```python
from build123d import *

# Parameters (mm, degrees)
SKETCH4_R           = 1.25
BOSS_EXTRUDE2_DEPTH = 5
CUT_EXTRUDE2_DEPTH  = 10


with BuildPart() as part:
    # Sketch4 → Boss-Extrude2 (new body)
    with BuildSketch(Plane(origin=(0, 0, 0), x_dir=(1, 0, 0), z_dir=(0, 1, 0))):
        Polygon((82.9, -82.75), (79, -82.75), (79, -86), (79, -88.5), (89, -88.5), (89, -80.85), (82.9, -80.85), align=None)
        with Locations((81.5, -86)):
            Circle(SKETCH4_R, mode=Mode.SUBTRACT)
    extrude(amount=BOSS_EXTRUDE2_DEPTH)

    # Sketch5 → Cut-Extrude2 (cut)
    with BuildSketch(Plane(origin=(89, 0, 0), x_dir=(0, 0, -1), z_dir=(1, 0, 0))):
        with BuildLine():
            ThreePointArc((-84.75, 3.75), (-86, 2.5), (-84.75, 1.25))
            Line((-84.75, 1.25), (-84.75, 3.75))
        make_face()
        with BuildLine():
            Line((-84.75, 3.75), (-84.75, 1.25))
            ThreePointArc((-84.75, 1.25), (-83.866116524, 1.616116524), (-83.5, 2.5))
            ThreePointArc((-83.5, 2.5), (-83.866116524, 3.383883476), (-84.75, 3.75))
        make_face()
    extrude(amount=-CUT_EXTRUDE2_DEPTH, mode=Mode.SUBTRACT)


solid = part.part
```
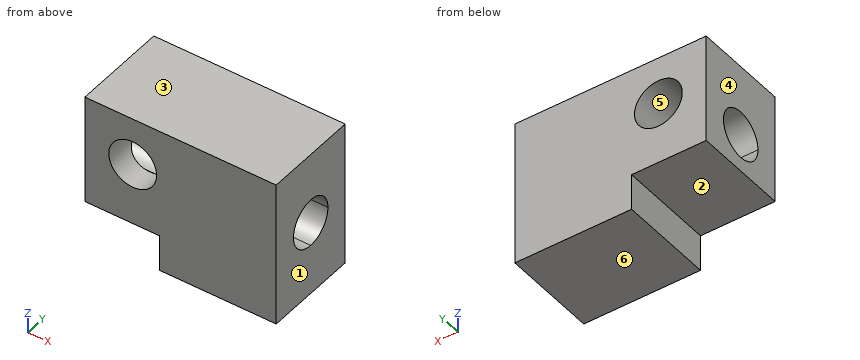
CAD build for the part. Positions are in the model's coordinates, mm. Face numbers are marked on the shaded views. A direction names the side the tool comes from. Round coordinates to 2 decimals unless told otherwise and drop trailing zeros. Write each loop counter-clockwise with the first axis right and the second up, starting at its lowest first coordinate (ties: lowest second). Pieces come first, ordered by that corner, then holes. Notation, with made-up numbers: M -23,25 L 28,25 A13 cw 28,50 Z; hole C -13.75,4 d11. An arc over 180 degrees is marked long. One line per question, with ' | ' between items.
1. Which spindle directions (+Z, -Z, +X, -X, +Y, -Y) get a long thin tool onto all of the face, cutting with end or side? Do the marked faces 1 and 2. Say none if no direction does.
Working result:
face 1: +Z, -Z, +X, +Y, -Y | face 2: -Z, -X, +Y, -Y
2. Cut at D-D on x = 80.75. Write the cut outline in (y, z).
Working result:
outline: M 0,82.75 L 5,82.75 L 5,85 L 3.72,85 A1.25 cw long 1.28,85 L 0,85 Z; M 0,87 L 5,87 L 5,88.5 L 0,88.5 Z
3. Cut at C-C on y = 4.7. Write the cut outline in (x, z).
Working result:
outline: M 79,82.75 L 82.9,82.75 L 82.9,80.85 L 89,80.85 L 89,88.5 L 79,88.5 Z; hole C 81.5,86 d2.5
4. Pin check, flat tip, straight feed: pin 1 Ø0.6 at (y, z) = (3, 82) entering from -X. Stop position of the tip, or through.
Working result:
pin 1: x = 82.9
5. Cut at A-A on x = 85.75. Write the cut outline in (y, z), and give its area (3 significant figures).
Working result:
outline: M 0,80.85 L 5,80.85 L 5,88.5 L 0,88.5 Z; hole C 2.5,84.75 d2.5 | area: 33.3 mm2
6. Probe L1, parallel to X at y = 3.35, z = 86; L2, parallel to Z at x = 81.5, y = 2.5; L3, parallel to Z at x = 81.5, y = 1. List the from-to ranges inside material, lowest first. Write a range as from..to.
Working result:
L1: 79..80.25, 82.75..89 | L2: 82.75..83.5, 87.25..88.5 | L3: 82.75..84.75, 87.25..88.5
7. Cut at B-B on z = 84. Write the cut outline in (x, y).
Working result:
outline: M 79,0 L 89,0 L 89,1.5 L 79,1.5 Z; M 79,3.5 L 89,3.5 L 89,5 L 79,5 Z
8. Mould opens along Z. For the marked faces 3, 4, 5 and 6 say: pulls with the +Z half, pulls with the -Z half, needs draft (parallel to the pull), parting line crosses it, or undercut.
Working result:
face 3: pulls with the +Z half | face 4: needs draft | face 5: undercut | face 6: pulls with the -Z half
